Drawing for the job (mm, zero at the part's lowest x, y, z). A direction names the side the tool comes from. Give positions to 0.01 mm unless a question says otherwise; leave off trailing zeros. Write each loop counter-clockwise with the first axis right and the second up, starting at its lowest first coordinate (ties: lowest second). Pieces come first, ordered by that corner, then holes.
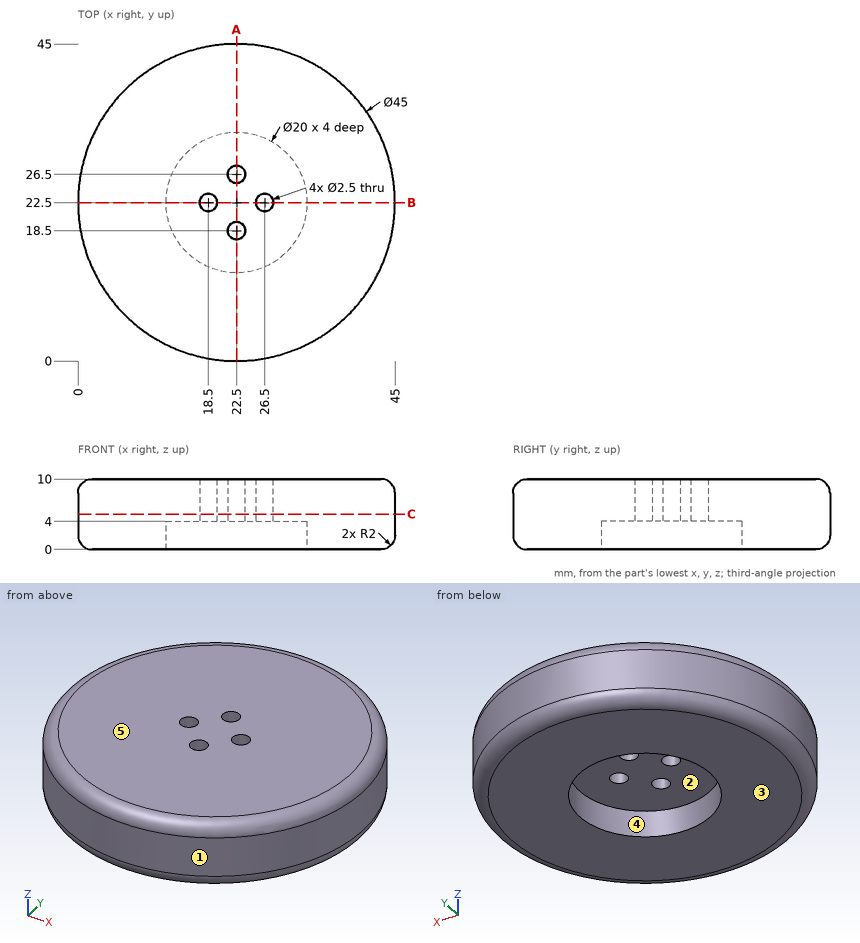
1. Pull direction Y, two halves, no side cores. Call the marked faces 1, 2 and 3: +Y half, -Y half, draft (parallel to the pull), parting line (faces both ways), or undercut.
Calculated:
face 1: parting line
face 2: undercut
face 3: draft
2. Slice it at A-A, the plane x = 22.5. Write the cut outline in (y, z), and give its area (3 significant figures).
Calculated:
outline: (0, 2) arc R2 ccw to (2, 0) - (12.5, 0) - (12.5, 4) - (17.25, 4) - (17.25, 10) - (2, 10) arc R2 ccw to (0, 8) - close; (19.75, 4) - (25.25, 4) - (25.25, 10) - (19.75, 10) - close; (27.75, 4) - (32.5, 4) - (32.5, 0) - (43, 0) arc R2 ccw to (45, 2) - (45, 8) arc R2 ccw to (43, 10) - (27.75, 10) - close
area: 337 mm2
3. Slice it at C-C, the plane z = 5. Write the cut outline in (x, y), and give its area (3 significant figures).
Calculated:
outline: circle Ø45 at (22.5, 22.5); hole circle Ø2.5 at (18.5, 22.5); hole circle Ø2.5 at (22.5, 18.5); hole circle Ø2.5 at (22.5, 26.5); hole circle Ø2.5 at (26.5, 22.5)
area: 1,570 mm2
4. Probe probe 1 along Y at (x, z) = (22.5, 6.2); probe 2 along Z at (x, y) = (18, 29.5); probe 3 along Y at (x, z) = (22, 3). List the from-to ranges inside material, lowest first.
Calculated:
probe 1: y = 0 to 17.25, 19.75 to 25.25, 27.75 to 45
probe 2: z = 4 to 10
probe 3: y = 0.01 to 12.51, 32.49 to 44.99
5. Pin check, flat tips, straight feed: P1, Ø5, axis at y = 32, z = 5.5, coming from the +X side; P2, Ø1, axis at y = 23.5, z = 6, coming from the -X side; P3, Ø4, axis at x = 27.5, y = 12.5, coming from the -Z side; P4, Ø3, axis at x = 29.5, z = 9, coming from the +Y side. Stop position of each tip, or through.
Calculated:
P1: stops at x = 43.88
P2: stops at x = 0.01
P3: stops at z = 0
P4: stops at y = 44.25
6. Which spindle directions (+Z, -Z, +X, -X, +Y, -Y) get a long thin tool onto all of the face, cutting with end or side? Do the marked faces 4 and 5. Say none if no direction does.
Calculated:
face 4: -Z
face 5: +Z, +X, -X, +Y, -Y
